Source: CAD feature listing. Evaluate the final solid. Frame: model axes, mm. Face numbers are marked on the shaded views. A direction names the side the tool comes from. Give positions to 0.01 mm unless a question says otherwise; leave off trailing zeros. Order: outer loops, then holes, each group sorted by start corner. A loop starts at its lowest first (then second) coordinate and runs counter-clockwise, first axis right, second up.
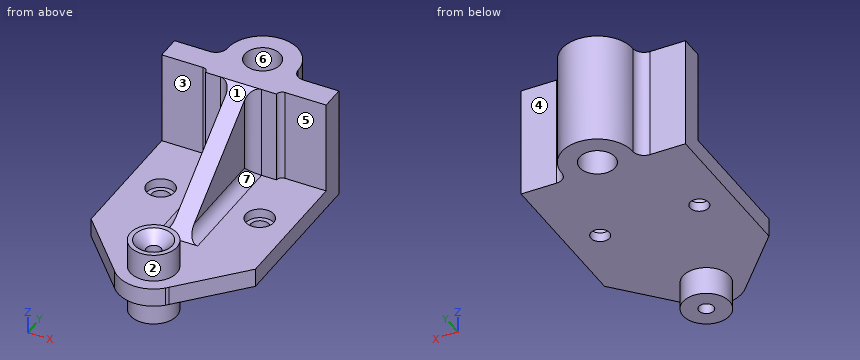
from build123d import *

# Parameters (mm, degrees)
SKETCH1_R           = 9.5
BOSS_EXTRUDE1_DEPTH = 60
BOSS_EXTRUDE2_DEPTH = 10
FILLET1_R           = 6
FILLET2_R           = 6
FILLET3_R           = 3
BOSS_EXTRUDE4_DEPTH = 5
FILLET4_R           = 6
FILLET5_R           = 6
SKETCH6_R           = 12.5
BOSS_EXTRUDE5_DEPTH = 20
HOLE2_D             = 8
HOLE2_DEPTH         = 39.547439867
HOLE2_CSINK_D       = 20
HOLE2_CSINK_ANGLE   = 90
CUT_EXTRUDE1_START  = -40
SKETCH13_R          = 4
CUT_EXTRUDE1_DEPTH  = 40
HOLE4_D             = 10
HOLE4_CBORE_D       = 15
HOLE4_CBORE_DEPTH   = 5


# Some blends are built 0.0001 mm under size
with BuildPart() as part:
    # Sketch1 → Boss-Extrude1 (new body)
    with BuildSketch(Plane.XY):
        with BuildLine():
            Line((0, 0), (38, 0))
            Line((38, 0), (38, 3))
            Line((38, 3), (63, 3))
            Line((63, 3), (63, 16))
            Line((63, 16), (38, 16))
            Line((38, 16), (38, 22))
            ThreePointArc((38, 22), (19, 41), (0, 22))
            Line((0, 22), (0, 16))
            Line((0, 16), (-25, 16))
            Line((-25, 16), (-25, 3))
            Line((-25, 3), (0, 3))
            Line((0, 3), (0, 0))
        make_face()
        with Locations((19, 22)):
            Circle(SKETCH1_R, mode=Mode.SUBTRACT)
    extrude(amount=BOSS_EXTRUDE1_DEPTH)

    # Sketch2 → Boss-Extrude2 (add)
    with BuildSketch(Plane.XY):
        with BuildLine():
            Line((63, -69), (63, 3))
            Line((63, 3), (38, 3))
            Line((38, 3), (38, 0))
            Line((38, 0), (19, 0))
            Line((19, 0), (0, 0))
            Line((0, 0), (0, 3))
            Line((0, 3), (-25, 3))
            Line((-25, 3), (-25, -69))
            Line((-25, -69), (4.520418495, -101.302102237))
            ThreePointArc((4.520418495, -101.302102237), (18.194672039, -107.98292514), (32.385626244, -102.484250445))
            Line((32.385626244, -102.484250445), (33.626524101, -101.127027365))
            Line((33.626524101, -101.127027365), (63, -69))
        make_face()
        with BuildLine():
            ThreePointArc((19, -101.5), (6.5, -89), (19, -76.5))
            ThreePointArc((19, -76.5), (27.838834765, -80.161165235), (31.5, -89))
            ThreePointArc((31.5, -89), (27.838834765, -97.838834765), (19, -101.5))
        make_face(mode=Mode.SUBTRACT)
    extrude(amount=BOSS_EXTRUDE2_DEPTH)

    # Fillet1
    fillet1_edges = [part.edges().sort_by_distance(p)[0] for p in [
        (0, 16, 30),
    ]]
    fillet(fillet1_edges, radius=FILLET1_R - 0.0001)  # a hair under: the kernel refuses the full size

    # Fillet2
    fillet2_edges = [part.edges().sort_by_distance(p)[0] for p in [
        (38, 16, 30),
    ]]
    fillet(fillet2_edges, radius=FILLET2_R - 0.0001)  # a hair under: the kernel refuses the full size

    # Fillet3
    fillet3_edges = [part.edges().sort_by_distance(p)[0] for p in [
        (0, 3, 35),
        (38, 3, 35),
    ]]
    fillet(fillet3_edges, radius=FILLET3_R - 0.0001)  # a hair under: the kernel refuses the full size

    # Sketch4 → Boss-Extrude4 (add, symmetric)
    with BuildSketch(Plane(origin=(19, 0, 0), x_dir=(0, 0, -1), z_dir=(1, 0, 0))):
        Polygon((-60, 0), (-10, -65), (-10, 0), align=None)
    extrude(amount=BOSS_EXTRUDE4_DEPTH, both=True)

    # Fillet4
    # the kernel refuses this fillet: 6 mm, written as the material it adds along each edge
    with BuildSketch(Plane(origin=(14, 0, -5), x_dir=(-1, 0, 0), z_dir=(0, 0, 1))) as fillet4_piece_1_section:
        with BuildLine():
            CenterArc((FILLET4_R, FILLET4_R), FILLET4_R, 180, 90)
            Line((0, FILLET4_R), (0, 0))
            Line((0, 0), (FILLET4_R, 0))
        make_face()
    fillet4_piece_1 = extrude(amount=80, mode=Mode.PRIVATE)
    fillet4_piece_1 = split(fillet4_piece_1, bisect_by=Plane(origin=(12.648095827, -13.156695973, 49.879464636), z_dir=(0, 0.6097107608496924, -0.7926239891046001)), keep=Keep.TOP, mode=Mode.PRIVATE)
    fillet4_piece_1 = split(fillet4_piece_1, bisect_by=Plane(origin=(12.648095827, -1.320325191, 0), z_dir=(0, 0, 1)), keep=Keep.TOP, mode=Mode.PRIVATE)
    add(fillet4_piece_1)
    with BuildSketch(Plane(origin=(24, 0, -5), x_dir=(1, 0, 0), z_dir=(0, 0, 1))) as fillet4_piece_2_section:
        with BuildLine():
            CenterArc((FILLET4_R, -FILLET4_R), FILLET4_R, 90, 90)
            Line((0, -FILLET4_R), (0, 0))
            Line((0, 0), (FILLET4_R, 0))
        make_face()
    fillet4_piece_2 = extrude(amount=80, mode=Mode.PRIVATE)
    fillet4_piece_2 = split(fillet4_piece_2, bisect_by=Plane(origin=(25.351904173, -13.156695973, 49.879464636), z_dir=(0, 0.6097107608496924, -0.7926239891046001)), keep=Keep.TOP, mode=Mode.PRIVATE)
    fillet4_piece_2 = split(fillet4_piece_2, bisect_by=Plane(origin=(25.351904173, -1.320325191, 0), z_dir=(0, 0, 1)), keep=Keep.TOP, mode=Mode.PRIVATE)
    add(fillet4_piece_2)

    # Fillet5
    # the kernel refuses this fillet: 6 mm, written as the material it adds along each edge
    with BuildSketch(Plane(origin=(24, -80, 10), x_dir=(1, 0, 0), z_dir=(0, 1, 0))) as fillet5_piece_1_section:
        with BuildLine():
            CenterArc((FILLET5_R, -FILLET5_R), FILLET5_R, 90, 90)
            Line((0, -FILLET5_R), (0, 0))
            Line((0, 0), (FILLET5_R, 0))
        make_face()
    fillet5_piece_1 = extrude(amount=89, mode=Mode.PRIVATE)
    fillet5_piece_1 = split(fillet5_piece_1, bisect_by=Plane(origin=(25.330544352, -46.320917546, 24.368524964), z_dir=(0, 0.6097107608496924, -0.7926239891046002)), keep=Keep.TOP, mode=Mode.PRIVATE)
    add(fillet5_piece_1)
    with BuildSketch(Plane(origin=(14, -80, 10), x_dir=(-1, 0, 0), z_dir=(0, 1, 0))) as fillet5_piece_2_section:
        with BuildLine():
            CenterArc((FILLET5_R, FILLET5_R), FILLET5_R, 180, 90)
            Line((0, FILLET5_R), (0, 0))
            Line((0, 0), (FILLET5_R, 0))
        make_face()
    fillet5_piece_2 = extrude(amount=89, mode=Mode.PRIVATE)
    fillet5_piece_2 = split(fillet5_piece_2, bisect_by=Plane(origin=(12.669455648, -46.320917546, 24.368524964), z_dir=(0, 0.6097107608496924, -0.7926239891046002)), keep=Keep.TOP, mode=Mode.PRIVATE)
    add(fillet5_piece_2)

    # Sketch6 → Boss-Extrude5 (add, symmetric)
    with BuildSketch(Plane.XY.offset(5)):
        with Locations((19, -89)):
            Circle(SKETCH6_R)
    extrude(amount=BOSS_EXTRUDE5_DEPTH, both=True)

    # Hole2
    with Locations(Plane.XY.offset(25)):
        with Locations((19, -89)):
            CounterSinkHole(HOLE2_D / 2, HOLE2_CSINK_D / 2, depth=HOLE2_DEPTH, counter_sink_angle=HOLE2_CSINK_ANGLE)

    # Sketch13 → Cut-Extrude1 (cut)
    with BuildSketch(Plane.XY.offset(-14.547439867).offset(CUT_EXTRUDE1_START)):
        with Locations((19, -89)):
            Circle(SKETCH13_R)
    extrude(amount=CUT_EXTRUDE1_DEPTH, mode=Mode.SUBTRACT)

    # Hole4 (through all)
    with Locations(Plane(origin=(-7.536351987, -31.351857419, 10), x_dir=(1, 0, 0), z_dir=(0, 0, 1))):
        with Locations((0, 0)):
            hole4 = CounterBoreHole(HOLE4_D / 2, HOLE4_CBORE_D / 2, HOLE4_CBORE_DEPTH)

    # Mirror2: Hole4 across plane
    add(hole4.mirror(Plane(origin=(19, 0, 0), x_dir=(0, 0, 1), z_dir=(1, 0, 0))), mode=Mode.SUBTRACT)


solid = part.part
1) First-contact query: pin 1 Ø1 at (x, y) = (26, 3) entering from -Z; pin 2 Ø1.5 at (x, y) = (25.5, -22) entering from +Z; pin 3 Ø4 at (x, z) = (34, 46.5) entering from -Y. Flat tips, straight axial feed; report the tip coordinate or a pass-through.
Checks:
pin 1: stops at z = 0
pin 2: stops at z = 13.1
pin 3: stops at y = 0
2) Ray query, L1, parallel to X at y = -89, z = -2.5; L2, parallel to Y at x = 24.5, z = 23; L3, parallel to Z at x = 34, y = -4.5. Return the intervals inside material, ascending.
Checks:
L1: x = 6.5 to 15, 23 to 31.5
L2: y = -100.22 to -94.81, -83.19 to -77.78, -3.6 to 14.25, 29.75 to 40.19
L3: z = 0 to 10
3) Section query D-D on y = -3. Output: boundary loops of the cut face in (x, z), and give its area (3 significant figures).
Checks:
outline: (-25, 0) - (63, 0) - (63, 10) - (30, 10) arc R6 cw to (24.8, 13) - (24.8, 57.69) - (13.2, 57.69) - (13.2, 13) arc R6 cw to (8, 10) - (-25, 10) - close
area: 1,440 mm2
4) Section query A-A on x = 19. Output: boundary loops of the cut face in (y, z).
Checks:
outline: (-108, 0) - (-101.5, 0) - (-101.5, -15) - (-93, -15) - (-93, 19) - (-99, 25) - (-101.5, 25) - (-101.5, 10) - (-108, 10) - close; (-85, -15) - (-76.5, -15) - (-76.5, 0) - (12.5, 0) - (12.5, 60) - (0, 60) - (-65, 10) - (-76.5, 10) - (-76.5, 25) - (-79, 25) - (-85, 19) - close; (31.5, 0) - (41, 0) - (41, 60) - (31.5, 60) - close
5) Reachability of the marked faces 1, 2, 3 and 4 from +Z, -Z, +X, -X, +Y, -Y: full face, straight path, thin tool, end or side. Return the list, or none.
Checks:
face 1: +Z, +X, -X
face 2: +Z
face 3: +Z, -X, -Y
face 4: +Z, -Z, +X, +Y
6) Section query C-C on y = 18.5. Output: boundary loops of the cut face in (x, z).
Checks:
outline: (-1.13, 0) - (10.17, 0) - (10.17, 60) - (-1.13, 60) - close; (27.83, 0) - (39.13, 0) - (39.13, 60) - (27.83, 60) - close
7) Pull-direction query (X, two-part tool) for the marked faces 5, 6 and 7; classes: +X half, -X half, draft (parallel to the pull), parting line (faces both ways), or undercut.
Checks:
face 5: draft
face 6: undercut
face 7: +X half
